```python
from build123d import *

# Parameters (mm, degrees)
F1_DEPTH = 63.5
F0_W     = 25.4
F0_H     = 19.05
F2_DEPTH = 25.4
F3_DEPTH = 8.255
F5_R     = 6.35
F6_R     = 1.27
F7_R     = 5.08


with BuildPart() as f1:
    # F0 (on Front) → F1 (new body, symmetric)
    with BuildSketch(Plane.XZ):
        Polygon((22.225, 9.525), (-41.275, 9.525), (-41.275, -9.525), (41.275, -9.525), (41.275, 9.525), align=None)
    extrude(amount=F1_DEPTH, both=True)

    # F0 (on Front) → F2 (join, symmetric)
    with BuildSketch(Plane.XZ):
        with Locations((80.6532034516, 53.8579252303)):
            Rectangle(F0_W, F0_H)
        with BuildLine():
            Line((22.225, 28.4579252303), (22.225, 9.525))
            Line((22.225, 9.525), (41.275, 9.525))
            Line((41.275, 9.525), (41.275, 28.4579252303))
            ThreePointArc((41.275, 28.4579252303), (45.9246798487, 39.6832453816), (57.15, 44.3329252303))
            Line((57.15, 44.3329252303), (67.9532034516, 44.3329252303))
            Line((67.9532034516, 44.3329252303), (67.9532034516, 63.3829252303))
            Line((67.9532034516, 63.3829252303), (57.15, 63.3829252303))
            ThreePointArc((57.15, 63.3829252303), (32.4542956671, 53.1536295632), (22.225, 28.4579252303))
        make_face()
    extrude(amount=F2_DEPTH, both=True)

    # F0 (on Front) → F3 (join, symmetric)
    with BuildSketch(Plane.XZ):
        with BuildLine():
            add(Edge.make_bspline(
                [(-41.275, 9.525), (-40.6863895337, 42.2286015016), (12.2434897348, 63.7291564518), (57.15, 63.3829252303)],
                knots=[0, 0, 0, 0, 112.1969551062, 112.1969551062, 112.1969551062, 112.1969551062], degree=3))
            Line((-41.275, 9.525), (22.225, 9.525))
            Line((22.225, 9.525), (22.225, 28.4579252303))
            ThreePointArc((22.225, 28.4579252303), (32.4542956671, 53.1536295632), (57.15, 63.3829252303))
        make_face()
    extrude(amount=F3_DEPTH, both=True)

    # F0 (on Front) → F4 (revolve)
    with BuildSketch(Plane.XZ):
        Polygon((93.3532034516, 66.675), (93.3532034516, 63.3829252303), (93.3532034516, 44.3329252303), (93.3532034516, 38.1), (118.7532034516, 38.1), (118.7532034516, 66.675), align=None)
    revolve(axis=Axis((93.3532034516, 0, 52.3875), (0, 0, 1)))

    # F5
    f5_edges = [f1.edges().sort_by_distance(p)[0] for p in [
        (41.275, -63.5, 0),
        (-41.275, -63.5, 0),
        (-41.275, 63.5, 0),
        (41.275, 63.5, 0),
    ]]
    fillet(f5_edges, radius=F5_R)

    # F6
    f6_edges = [f1.edges().sort_by_distance(p)[0] for p in [
        (67.953203, 0, 66.675),
    ]]
    fillet(f6_edges, radius=F6_R)

    # F7
    f7_edges = [f1.edges().sort_by_distance(p)[0] for p in [
        (67.953203, 0, 38.1),
    ]]
    fillet(f7_edges, radius=F7_R)


solid = f1.part
```
Work out the finished part from the listing and answer in its coordinate system (mm). A direction names the side the tool comes from. Round coordinates to 2 decimals unless told otherwise and drop trailing zeros. Order: outer loops, then holes, each group sorted by start corner. A loop starts at its lowest first (then second) coordinate and runs counter-clockwise, first axis right, second up.
Q1. A cutting plane is placed at A-A, the plane y = 49. Determine the outline of the cut face in (x, z) (3 decimals), then the cut area to 3 significant figures.
Solution:
outline: (-41.275, -9.525) - (41.275, -9.525) - (41.275, 9.525) - (-41.275, 9.525) - close
area: 1,570 mm2
Q2. A tool of negligible diameter and unlimited length cuts with its end or side. For faces 5 (the flat face through (49, -25.4, 43)), 6 (the flat face through (41.275, -1, 5)), 7 (the flat face through (49, 25.4, 43)), 8 (the flat face through (-2, -8.255, 31)), 9 (the cylindrical face through (32.727, 16.707, 53.424)), from which of +Z, -Z, +X, -X, +Y, -Y can it reach the whole face along a straight path? Write none if from no direction.
Solution:
face 5: +Z, +X, -X, -Y
face 6: -Z, +X, +Y, -Y
face 7: +Z, +X, -X, +Y
face 8: +Z, -X, -Y
face 9: +Z, -X, +Y
Q3. Given pin 1 Ø1 at (x, y) = (29, -47.5) entering from +Z (3 decimals); pin 2 Ø6 at (y, z) = (7.5, 32.5) entering from +X; pin 3 Ø18 at (x, y) = (70, 12) entering from +Z (3 decimals); pin 4 Ø5 at (y, z) = (21, 23) entering from -X (3 decimals), each flat-ended and moving along its own axis, determine where each tip first touches the part or whether it passes through.
Solution:
pin 1: stops at z = 9.525
pin 2: stops at x = 42.92
pin 3: stops at z = 66.675
pin 4: stops at x = 22.225
Q4. The mould has two halves that part along X. Classify faces 1 (the flat face through (67, 0, 44.333)), 2 (the flat face through (0, -63.5, 0)), 3 (the cylindrical face through (39.464, 61.59, 0.133)), 4 (the cylindrical face through (45.8, -0.36, 39.56)): pulls with the +X half, pulls with the -X half, needs draft (parallel to the pull), parting line crosses it, or undercut.
Solution:
face 1: undercut
face 2: needs draft
face 3: pulls with the +X half
face 4: undercut
Q5. Find the intervals of material crossed by line 1 along Z through (x, y) = (84, 18) (3 decimals); line 2 along Z through (x, y) = (11, 22) (3 decimals); line 3 along Y through (x, z) = (5, 40.5) (3 decimals), in increasing order.
Solution:
line 1: z = 38.1 to 66.675
line 2: z = -9.525 to 9.525
line 3: y = -8.255 to 8.255
